Model file for the job. Use its own axes, mm. Face numbers are marked on the shaded views. A direction names the side the tool comes from. Round coordinates to 2 decimals unless told otherwise and drop trailing zeros. Loops run counter-clockwise (first coordinate to the right, second up) from the corner with the lowest first, then second, coordinate; pieces in that order, holes last. Notation, with made-up numbers: (36.25, 78.5) -> (89.25, 78.5) arc R9 cw to (89.25, 82.5) -> close; hole circle Ø11 at (49.25, 45.5). An arc over 180 degrees is marked (long way). Use a Markdown table: item, result. Add a question column.
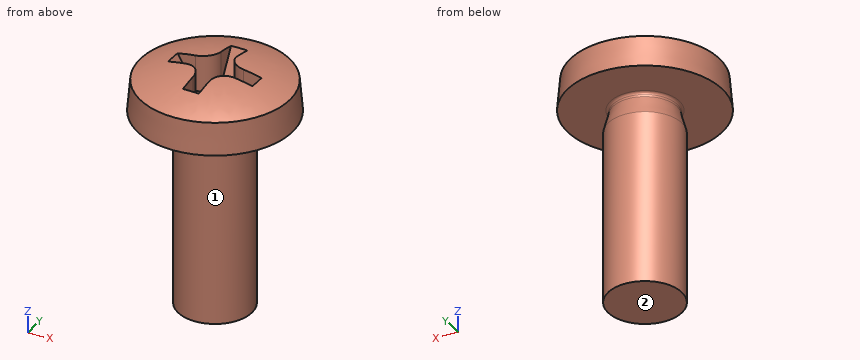
Autodesk Fusion 360 part; units mm, degrees
sketch "Sketch1" plane through (0, 0, 0) normal (0, 1, 0) x (1, 0, 0)
  line L0 (0, -1.9) -> (0, 8)
  line L1 (-3.15, 0) -> (-3.0363, -1.3)
  line L2 (-3.15, 0) -> (-1.299, 0)
  arc A0 (-3.0363, -1.3) -> (0, -1.9) centre (0, 6.0824) ccw
  line L3 (0, 8) -> (-1.5, 8)
  line L4 (-1.5, 8) -> (-1.5, 0.94)
  line L5 (-1.5, 0.94) -> (-1.299, 0.19)
  line L6 (-1.299, 0.19) -> (-1.299, 0)
  dimension "d13" = 5
  dimension "d14" = 6.3
  dimension "d18" = 3
  dimension "d23" = 15
  dimension "d53" = 1.9
  dimension "d55" = 7.06
  dimension "d56" = 8
  dimension "d57" = 7.81
  dimension "d60" = 1.3
revolve "Revolve1" add sketch "Sketch1" angle 360 about axis through (0, 0, 1.9) along (0, 0, -1) makes body 1
fillet "Fillet2" radius 0.1 1 edges at (-1.2111, 0.4698, 0) on bodies 1
ref_plane "WorkPlane1" through (0, 0, 1.9) normal (0, 0, 1) x (1, 0, 0)
sketch "Sketch2" plane through (0, 0, 1.9) normal (0, 0, 1) x (1, 0, 0)
  line L0 (-1.85, 0) -> (1.85, 0) construction
  line L1 (0, -1.85) -> (0, 1.85) construction
  line L2 (-0.331, 1.85) -> (0.331, 1.85)
  line L3 (0.331, 1.85) -> (0.331, 0.331)
  line L4 (0.331, 0.331) -> (1.85, 0.331)
  line L5 (1.85, 0.331) -> (1.85, -0.331)
  line L6 (1.85, -0.331) -> (0.331, -0.331)
  line L7 (0.331, -0.331) -> (0.331, -1.85)
  line L8 (0.331, -1.85) -> (-0.331, -1.85)
  line L9 (-0.331, -1.85) -> (-0.331, -0.331)
  line L10 (-0.331, -0.331) -> (-1.85, -0.331)
  line L11 (-1.85, -0.331) -> (-1.85, 0.331)
  line L12 (-1.85, 0.331) -> (-0.331, 0.331)
  line L13 (-0.331, 0.331) -> (-0.331, 1.85)
  dimension "d58" = 0.662
  dimension "d59" = 0.662
  dimension "d61" = 3.7
  dimension "d62" = 3.7
extrude "Extrude1" add sketch "Sketch2" against normal blind 1.53 separate body makes body 2
draft "Draft1" angle -30 neutral plane through (0, 0, 1.9) pull (0, 0, 1) 4 faces at (0.1103, -1.85, 1.39) (-0.1103, 1.85, 1.39) (-1.85, -0.1103, 1.39) (1.85, 0.1103, 1.39) on bodies 2
fillet "Fillet1" radius 0.662 4 edges at (0.331, -0.331, 1.135) (-0.331, -0.331, 1.135) (-0.331, 0.331, 1.135) (0.331, 0.331, 1.135) on bodies 2
combine "Combine1" operation cut target body 1 tool bodies 2
thread "Thread1" thread offset 0 thread length 10
equation "adsk_nomdia = 3.00 mm"
equation "adsk_nomlen = 8.00 mm"
equation "adsk_headdia = 6.30 mm"
equation "adsk_baseh = 1.30 mm"
equation "adsk_phildia = 3.70 mm"
equation "adsk_midfillet = 0.10 mm"
equation "adsk_thrlen = 7.06 mm"
equation "adsk_phildepth = 1.53 mm"
equation "adsk_thrrun = 0.75 mm"
equation "adsk_thrang = 15.00 deg"
equation "adsk_headang = 5.00 deg"
equation "d13 = adsk_headang"
equation "d14 = adsk_headdia"
equation "adsk_ovalh = 0.60 mm"
equation "d18 = adsk_nomdia"
equation "d23 = adsk_thrang"
equation "d32 = adsk_baseh + adsk_ovalh"
equation "adsk_philwidth = 0.662 mm"
equation "d48 = adsk_philwidth"
equation "d52 = adsk_midfillet"
equation "d53 = adsk_baseh + adsk_ovalh"
equation "d55 = adsk_thrlen"
equation "d56 = adsk_nomlen"
equation "d57 = adsk_thrlen + adsk_thrrun"
equation "d58 = adsk_philwidth"
equation "d59 = adsk_philwidth"
equation "d60 = adsk_baseh"
equation "d61 = adsk_phildia"
equation "d62 = adsk_phildia"
properties part number "BHS JIS B 1111 - M3x8 Steel 4.6 Plain"
1) Tool access for the marked faces 1 and 2: list every direction of +Z, -Z, +X, -X, +Y, -Y with a clear straight run to the whole face (end or side of a thin tool).
2) Pin check, flat tips, straight feed: pin 1 Ø2 at (x, z) = (-0.5, -3) entering from -Y; pin 2 Ø1.5 at (x, z) = (-0.5, -3.5) entering from +Y; pin 3 Ø0.8 at (x, z) = (1.5, 1.5) entering from -Y; pin 4 Ø2 at (x, y) = (0, 0) entering from +Z. Stop position of each tip, or through.
3) Cut at A-A on z = -1.25. Write the cut outline in (x, y), and give its area (3 significant figures).
4) Wall check: probe 1 along Y at (x, z) = (0, -3.75); probe 2 along Y at (x, z) = (1.5, 1); probe 3 along Y at (x, z) = (-0.5, 0.5). Give the ranges that are in metal, low to high. Write a range as from..to.
Established:
| question | item | result |
|---|---|---|
| 1 | face 1 | -Z |
| 1 | face 2 | -Z, +X, -X, +Y, -Y |
| 2 | pin 1 | stops at y = -1.5 |
| 2 | pin 2 | stops at y = 1.5 |
| 2 | pin 3 | stops at y = -2.81 |
| 2 | pin 4 | stops at z = 1.87 |
| 3 | outline | circle Ø3 at (0, 0) |
| 3 | area | 7.07 mm^2 |
| 4 | probe 1 | y = -1.5..1.5 |
| 4 | probe 2 | y = -2.67..2.67 |
| 4 | probe 3 | y = -3.07..-0.55, 0.55..3.07 |
